Answer from the drawing. Dimensions are ordinates in mm from the lowest x, y and z of the part. A direction names the side the tool comes from. Give positions to 0.01 mm unless a question says otherwise; leave off trailing zeros. Loops run counter-clockwise (first coordinate to the right, second up) from the corner with the lowest first, then second, coordinate; pieces in that order, holes last. Notation, with made-up numbers: (81, 57) -> (126, 57) arc R34 cw to (126, 91) -> close; hole circle Ø9 at (29, 28.25). An arc over 180 degrees is marked (long way). Return JSON: item names as keys, results as strings. Group by question number.
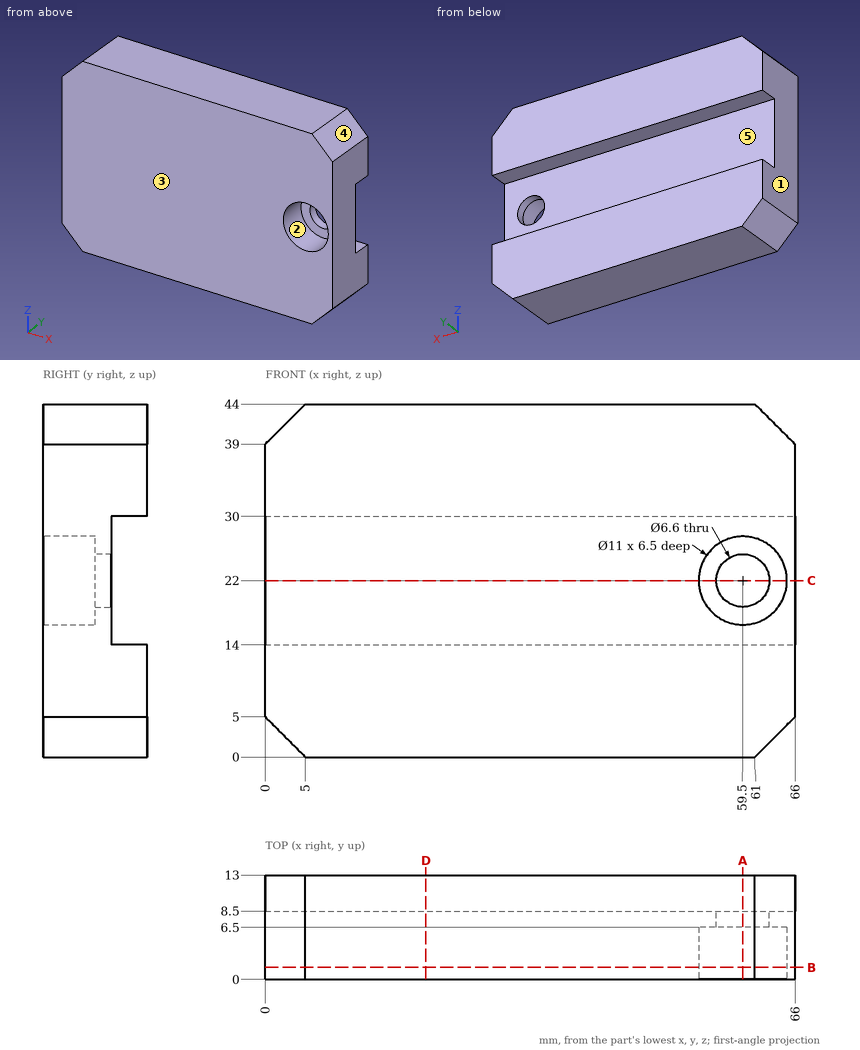
1. A flat-ended cylindrical pin translates along its axis: pin 1 Ø2 at (x, y) = (57, 3) entering from -Z. Find the tip coordinate at first contact, or state that the pin passes through.
2. Straight lines are drawn through the part: line 1 (Z direction, x = 29.5, y = 10.75); line 2 (X direction, y = 7.1, z = 22); line 3 (X direction, y = 1.5, z = 22). For each, find the intervals that lie inside material, in ascending order. Write a range as from..to.
3. Section B-B on y = 1.5 is taken. Determine the outline of the cut face in (x, z).
4. Section D-D on x = 20 is taken. Determine the outline of the cut face in (y, z), then the cut area to 3 significant figures.
5. Determine the mould class of the marked faces 3, 4 and 5 for opening direction Z: pulls with the +Z half, pulls with the -Z half, needs draft (parallel to the pull), parting line crosses it, or undercut.
6. Which of the six approach directions +Z, -Z, +X, -X, +Y, -Y give full straight-line access (tool end or side, diameter ignored) to the marked faces 1 and 2?
7. Section A-A on x = 59.5 is taken. Determine the outline of the cut face in (y, z).
8. Section C-C on z = 22 is taken. Determine the outline of the cut face in (x, y).
Completed:
{
 "1": {"pin 1": "stops at z = 0"},
 "2": {"line 1": "z = 0..14, 30..44", "line 2": "x = 0..56.2, 62.8..66", "line 3": "x = 0..54, 65..66"},
 "3": {"outline": "(0, 5) -> (5, 0) -> (61, 0) -> (66, 5) -> (66, 39) -> (61, 44) -> (5, 44) -> (0, 39) -> close; hole circle Ø11 at (59.5, 22)"},
 "4": {"outline": "(0, 0) -> (13, 0) -> (13, 14) -> (8.5, 14) -> (8.5, 30) -> (13, 30) -> (13, 44) -> (0, 44) -> close", "area": "500 mm²"},
 "5": {"face 3": "needs draft", "face 4": "pulls with the +Z half", "face 5": "undercut"},
 "6": {"face 1": "+Z, -Z, -X, +Y, -Y", "face 2": "-Y"},
 "7": {"outline": "(0, 0) -> (13, 0) -> (13, 14) -> (8.5, 14) -> (8.5, 18.7) -> (6.5, 18.7) -> (6.5, 16.5) -> (0, 16.5) -> close; (0, 27.5) -> (6.5, 27.5) -> (6.5, 25.3) -> (8.5, 25.3) -> (8.5, 30) -> (13, 30) -> (13, 44) -> (0, 44) -> close"},
 "8": {"outline": "(0, 0) -> (54, 0) -> (54, 6.5) -> (56.2, 6.5) -> (56.2, 8.5) -> (0, 8.5) -> close; (62.8, 6.5) -> (65, 6.5) -> (65, 0) -> (66, 0) -> (66, 8.5) -> (62.8, 8.5) -> close"}
}
